Drawing for the job (mm, zero at the part's lowest x, y, z). Give positions to 0.01 mm unless a question says otherwise; leave off trailing zeros. Loops run counter-clockwise (first coordinate to the right, second up) from the corner with the lowest first, then second, coordinate; pieces in that order, holes last.
1) Band-saw the part on C-C on z = 387.5. List the corners of the cut face in (x, y).
2) Flat gauge pins, fed straight in: P1, Ø6, axis at x = 126.5, y = 128, coming from the +Z side; P2, Ø5, axis at x = 93.5, y = 225, coming from the -Z side; P3, Ø6, axis at y = 86, z = 773.5, coming from the +X side; P4, Ø2, axis at x = 99.5, z = 462, coming from the +Y side. Where does each tip first touch, or does it go through?
3) Band-saw the part on A-A on y = 125. List the corners of the cut face in (x, z), then the cut area to 3 significant figures.
4) Wall check: line 1 (Y direction, x = 125, z = 768); line 2 (X direction, y = 188, z = 822); line 3 (X direction, y = 39.5, z = 547). Give the ranges that are in metal, low to high.
5) Band-saw the part on D-D on z = 527.5. List the corners of the cut face in (x, y), then the cut area to 3 significant figures.
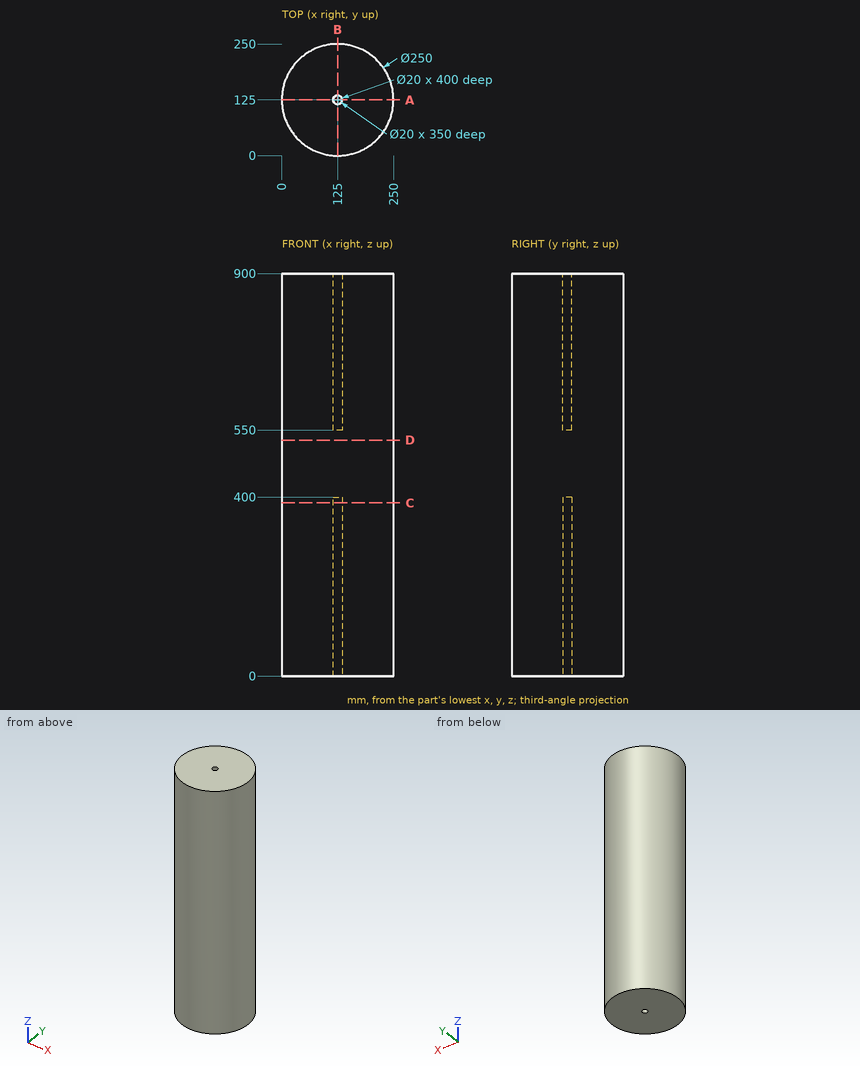
Findings below:
1. outline: circle Ø250 at (125, 125); hole circle Ø20 at (125, 125)
2. P1: stops at z = 550
2. P2: stops at z = 0
2. P3: stops at x = 244.7
2. P4: stops at y = 247.58
3. outline: (0, 0) - (115, 0) - (115, 400) - (135, 400) - (135, 0) - (250, 0) - (250, 900) - (135, 900) - (135, 550) - (115, 550) - (115, 900) - (0, 900) - close
3. area: 210,000 mm2
4. line 1: y = 0 to 115, 135 to 250
4. line 2: x = 17.04 to 232.96
4. line 3: x = 33.81 to 216.19
5. outline: circle Ø250 at (125, 125)
5. area: 49,100 mm2
